```python
from build123d import *

# Parameters (mm, degrees)
BOSS_EXTRUDE1_DEPTH = 15
FILLET1_R           = 7
SKETCH2_R           = 1
CUT_EXTRUDE1_DEPTH  = 8


with BuildPart() as part:
    # Sketch1 → Boss-Extrude1 (new body)
    with BuildSketch(Plane.XY):
        with BuildLine():
            Line((96.814228499, 422.253610621), (101.396155955, 422.253610621))
            ThreePointArc((101.396155955, 422.253610621), (112.002757673, 426.647008903), (116.396155955, 437.253610621))
            Line((116.396155955, 437.253610621), (116.396155955, 525.576232013))
            Line((116.396155955, 525.576232013), (124.396155955, 525.576232013))
            Line((124.396155955, 525.576232013), (124.396155955, 437.253610621))
            ThreePointArc((124.396155955, 437.253610621), (119.618915568, 423.220398868), (107.271718381, 415.016754589))
            Line((107.271718381, 415.016754589), (96.814228499, 412.253610621))
            Line((96.814228499, 412.253610621), (96.814228499, 422.253610621))
        make_face()
    extrude(amount=-BOSS_EXTRUDE1_DEPTH)

    # Fillet1
    fillet1_edges = [part.edges().sort_by_distance(p)[0] for p in [
        (120.396155955, 525.576232013, -15),
        (120.396155955, 525.576232013, 0),
    ]]
    fillet(fillet1_edges, radius=FILLET1_R)

    # Sketch2 → Cut-Extrude1 (cut)
    with BuildSketch(Plane.ZY.offset(-116.396155955)):
        with Locations((-7.5, 518.676232013)):
            Circle(SKETCH2_R)
    extrude(amount=-CUT_EXTRUDE1_DEPTH, mode=Mode.SUBTRACT)


solid = part.part
```
Geometry check sheet. Reference: the model listing, model coordinates, mm. A direction names the side the tool comes from. Coordinates: 2 decimals unless noted, no trailing zeros. Loops run counter-clockwise (first coordinate to the right, second up) from the corner with the lowest first, then second, coordinate; pieces in that order, holes last.
Item 1: Sectioned sample at A-A, the plane z = -12. Record the boundary of the cut face in (x, y).
Item 2: Thickness scan on line 1 (X direction, y = 516.5, z = -2); line 2 (Y direction, x = 120.25, z = -7.5); line 3 (Y direction, x = 122.5, z = -7.5). Record the ranges inside material, lowest first.
Item 3: Sectioned sample at B-B, the plane y = 465.5. Record the boundary of the cut face in (x, z), then the cut area to 3 significant figures.
Item 4: Sectioned sample at D-D, the plane x = 108.5. Record the boundary of the cut face in (y, z), then the cut area to 3 significant figures.
Item 5: Access from +Z, -Z, +X, -X, +Y, -Y to the whole of each face (thin tool, end or side, straight path). Record for faces 1 (the face through (120.452, 523.58, -2.105)), 2 (the face through (99, 422.254, -7)).
Item 6: Sectioned sample at C-C, the plane x = 117.5. Record the boundary of the cut face in (y, z).
Item 7: Go/stop test with flat-tipped pins: pin 1 Ø5 at (x, z) = (98, -8.5) entering from +Y; pin 2 Ø7.5 at (y, z) = (461.5, -5) entering from -X; pin 3 Ø1 at (x, z) = (105, -13) entering from -Y. Record where each tip stops, or that it passes through.
Item 8: Release check for a two-part mould opening along Y. For faces 3 (the face through (120.34, 517.79, -7.04)), 4 (the face through (116.396, 481, -7)), 5 (the face through (119.75, 423.39, -7.4)), 6 (the face through (120.452, 523.58, -12.895)) record: released by +Y, released by -Y, zero draft, split by the parting line, or undercut.
Check result:
1. outline: (96.81, 412.25) - (107.27, 415.02) arc R23 ccw to (124.4, 437.25) - (124.4, 524.32) - (116.4, 524.32) - (116.4, 437.25) arc R15 cw to (101.4, 422.25) - (96.81, 422.25) - close
2. line 1: x = 116.4 to 124.4
2. line 2: y = 424.08 to 517.68, 519.68 to 525.58
2. line 3: y = 428.11 to 517.68, 519.68 to 525.58
3. outline: (116.4, -15) - (124.4, -15) - (124.4, 0) - (116.4, 0) - close
3. area: 120 mm2
4. outline: (415.38, -15) - (424.04, -15) - (424.04, 0) - (415.38, 0) - close
4. area: 130 mm2
5. face 1: +Z, +X, -X, +Y
5. face 2: +Z, -Z, -X, +Y
6. outline: (420.83, -15) - (518.58, -15) arc R7 ccw to (525.58, -8) - (525.58, -7) arc R7 ccw to (518.58, 0) - (420.83, 0) - close; hole circle Ø2 at (518.68, -7.5)
7. pin 1: stops at y = 422.25
7. pin 2: stops at x = 116.4
7. pin 3: stops at y = 414.28
8. face 3: undercut
8. face 4: zero draft
8. face 5: released by -Y
8. face 6: released by +Y
